from build123d import *

# Parameters (mm, degrees)
SKIZZE1_R                       = 1.6
AUFSATZ_LINEAR_AUSTRAGEN1_DEPTH = 5


with BuildPart() as part:
    # Skizze1 → Aufsatz-Linear austragen1 (new body)
    with BuildSketch(Plane.XY):
        Polygon((5, 10), (5, 20), (0, 20), (0, 30), (5, 30), (5, 40), (0, 40), (0, 50), (5, 50), (5, 60), (0, 60), (0, 70), (5, 70), (5, 80), (0, 80), (0, 90), (5, 90), (5, 100), (0, 100), (0, 110), (5, 110), (5, 120), (0, 120), (0, 130), (5, 130), (5, 140), (0, 140), (0, 150), (5, 150), (5, 160), (0, 160), (0, 170), (5, 170), (5, 180), (0, 180), (0, 190), (5, 190), (5, 200), (0, 200), (0, 210), (5, 210), (5, 220), (35, 250), (45, 250), (45, 255), (55, 255), (55, 250), (65, 250), (65, 255), (75, 255), (75, 250), (85, 250), (85, 255), (95, 255), (95, 250), (105, 250), (105, 255), (115, 255), (115, 250), (125, 250), (125, 255), (135, 255), (135, 250), (145, 250), (145, 255), (155, 255), (155, 250), (165, 250), (165, 255), (175, 255), (175, 250), (185, 250), (185, 255), (195, 255), (195, 250), (205, 250), (205, 255), (215, 255), (215, 250), (225, 250), (225, 255), (235, 255), (235, 250), (245, 250), (245, 255), (255, 255), (255, 250), (265, 250), (265, 255), (275, 255), (275, 250), (305, 220), (305, 210), (310, 210), (310, 200), (305, 200), (305, 190), (310, 190), (310, 180), (305, 180), (305, 170), (310, 170), (310, 160), (305, 160), (305, 150), (310, 150), (310, 140), (305, 140), (305, 130), (310, 130), (310, 120), (305, 120), (305, 110), (310, 110), (310, 100), (305, 100), (305, 90), (310, 90), (310, 80), (305, 80), (305, 70), (310, 70), (310, 60), (305, 60), (305, 50), (310, 50), (310, 40), (305, 40), (305, 30), (310, 30), (310, 20), (305, 20), (305, 10), (310, 10), (310, 0), (305, 0), (305, -10), (310, -10), (310, -20), (305, -20), (305, -30), (310, -30), (310, -40), (305, -40), (305, -50), (310, -50), (310, -60), (305, -60), (305, -70), (310, -70), (310, -80), (305, -80), (5, -80), (0, -80), (0, -70), (5, -70), (5, -60), (0, -60), (0, -50), (5, -50), (5, -40), (0, -40), (0, -30), (5, -30), (5, -20), (0, -20), (0, -10), (5, -10), (5, 0), (0, 0), (0, 10), align=None)
        with Locations((20, 215)):
            Circle(SKIZZE1_R, mode=Mode.SUBTRACT)
        with Locations((30, 215)):
            Circle(SKIZZE1_R, mode=Mode.SUBTRACT)
        with Locations((290, 215)):
            Circle(SKIZZE1_R, mode=Mode.SUBTRACT)
        with Locations((280, 215)):
            Circle(SKIZZE1_R, mode=Mode.SUBTRACT)
    extrude(amount=AUFSATZ_LINEAR_AUSTRAGEN1_DEPTH)


solid = part.part
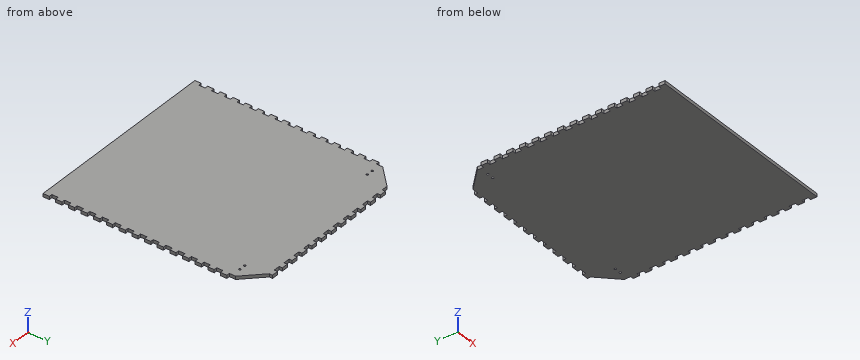
The listing builds one solid part. Answer for the finished solid, in the listing's coordinates (mm). Give positions to 0.01 mm unless a question says otherwise; leave off trailing zeros. Order: outer loops, then holes, each group sorted by start corner. A loop starts at its lowest first (then second) coordinate and runs counter-clockwise, first axis right, second up. Notation, with made-up numbers: (-37.5, 46) - (0.5, 46) arc R13 ccw to (0.5, 66) - close; hole circle Ø5 at (-36.75, 46). An arc over 180 degrees is marked (long way). Answer as CSV lines item,"result".
Q1. A cutting plane is placed at B-B, the plane y = 228. Determine the outline of the cut face in (x, z).
Answer key:
outline,"(13, 0) - (297, 0) - (297, 5) - (13, 5) - close"
Q2. Straight lines are drawn through the part: L1, parallel to X at y = 215, z = 2.85; L2, parallel to Y at x = 280, z = 2.95; L3, parallel to Y at x = 199, z = 2.6. For each, find the intervals that lie inside material, in ascending order.
Answer key:
L1,"x = 5 to 18.4, 21.6 to 28.4, 31.6 to 278.4, 281.6 to 288.4, 291.6 to 305"
L2,"y = -80 to 213.4, 216.6 to 245"
L3,"y = -80 to 250"
Q3. A cutting plane is placed at A-A, the plane z = 1.65. Count the separate pieces of the cut face and the enclosed holes in it, and give its area (3 significant figures).
Answer key:
separate pieces,"1"
enclosed holes,"4"
area,"100,000 mm^2"
Q4. Each of these flat-tipped pins is pushed along its axis until it touches: pin 1 Ø1.5 at (y, z) = (56.5, 1.5) entering from -X; pin 2 Ø2.5 at (x, y) = (290, 215) entering from +Z; pin 3 Ø12 at (x, y) = (44.5, -36.5) entering from -Z; pin 4 Ø2.5 at (y, z) = (175.5, 2) entering from +X. Where does it stop, or does it pass through?
Answer key:
pin 1,"stops at x = 5"
pin 2,"passes through"
pin 3,"stops at z = 0"
pin 4,"stops at x = 305"
